```python
from build123d import *

# Parameters (mm, degrees)
F0_W          = 210
F0_H          = 250
F1_DEPTH      = 0.5
F2_R          = 5.125
F2_R_2        = 4.125
F3_DEPTH      = 105
F3_DEPTH_BACK = 105


with BuildPart() as f1:
    # F0 (on Top) → F1 (new body, symmetric)
    with BuildSketch(Plane.XY):
        Rectangle(F0_W, F0_H)
    extrude(amount=F1_DEPTH, both=True)

    # F2 (on Right) → F3 (join, two sides)
    with BuildSketch(Plane.YZ) as f3_sk:
        with Locations((-130.100551, 0)):
            Circle(F2_R)
        with Locations((-130.100551, 0)):
            Circle(F2_R_2, mode=Mode.SUBTRACT)
    extrude(amount=F3_DEPTH)
    extrude(f3_sk.sketch, amount=-F3_DEPTH_BACK)

    # F4: F1 across plane


with BuildPart() as f1_1:
    add(f1.part)
    add(f1.part.mirror(Plane.XZ))


solid = f1_1.part
```
Input: part model. Units: mm. Frame: model coordinates. A direction names the side the tool comes from. Round coordinates to 2 decimals unless told otherwise and drop trailing zeros. Loops run counter-clockwise (first coordinate to the right, second up) from the corner with the lowest first, then second, coordinate; pieces in that order, holes last. Notation, with made-up numbers: (69, -20.5) -> (115, -20.5) arc R18 ccw to (115, -8.5) -> close; hole circle Ø7 at (-26, 16). An arc over 180 degrees is marked (long way). One line per item, written item: value.
(1) Material intervals for line 1 (Y direction, x = 64, z = -0.75); line 2 (Y direction, x = 35, z = -3.5); line 3 (Y direction, x = -95, z = 0.25), sorted ascending. Write a range as [from, to].
Geometry check:
line 1: [-135.17, -134.16], [-126.04, -125.03], [125.03, 126.04], [134.16, 135.17]
line 2: [-133.84, -132.28], [-127.92, -126.36], [126.36, 127.92], [132.28, 133.84]
line 3: [-135.22, -134.22], [-125.98, 125.98], [134.22, 135.22]
(2) Set-up query: faces 4 (the face through (-1, 2, 0.5)), 5 (the face through (-1, 2, -0.5)), 6 (the face through (1.47, -135.22, 0.22)). Return all of +Z, -Z, +X, -X, +Y, -Y with unobstructed straight access to the full face (end or side cutting, diameter ignored); none if empty.
Geometry check:
face 4: +Z, +X, -X
face 5: -Z, +X, -X
face 6: +X, -X
(3) Section B-B (y = 31). Return the cut outline in (x, z).
Geometry check:
outline: (-105, -0.5) -> (105, -0.5) -> (105, 0.5) -> (-105, 0.5) -> close
(4) Section A-A (x = 9). Return the cut outline in (y, z) (3 decimals).
Geometry check:
outline: (-125, -0.5) -> (125, -0.5) arc R5.125 ccw (long way) to (125, 0.5) -> (-125, 0.5) arc R5.125 ccw (long way) to start; hole circle Ø8.25 at (-130.101, 0); hole circle Ø8.25 at (130.101, 0)
(5) Pin query (flat end, axial travel): pin 1 (1 mm diameter, centred on x = -55.5, z = -1, fed in from +Y); pin 2 (2 mm diameter, centred on x = -80, y = 39, fed in from +Z); pin 3 (2 mm diameter, centred on y = -54, z = 2, fed in from -X); pin 4 (1.5 mm diameter, centred on x = 28, y = -77.5, fed in from -Z). Return the tip coordinate at first contact, or that it passes through.
Geometry check:
pin 1: y = 135.2
pin 2: z = 0.5
pin 3: through
pin 4: z = -0.5
(6) Mould query, pull axis Y, two halves, no side actions, for faces 1 (the face through (1.47, 135.22, 0.22)), 2 (the face through (-105, 1, 0)), 3 (the face through (1.47, 134.22, 0.18)). Classes: pulls with the +Y half, pulls with the -Y half, needs draft (parallel to the pull), parting line crosses it, or undercut.
Geometry check:
face 1: undercut
face 2: needs draft
face 3: undercut
